Geometry: final body of the model. Coordinates: model frame, mm. Face numbers are marked on the shaded views. A direction names the side the tool comes from. Coordinates: 2 decimals unless noted, no trailing zeros. Loops run counter-clockwise (first coordinate to the right, second up) from the corner with the lowest first, then second, coordinate; pieces in that order, holes last. Notation, with made-up numbers: (60, -5) - (102, -5) arc R9 ccw to (102, 1) - close; hole circle Ø10 at (84, 68.25). An arc over 180 degrees is marked (long way). Return JSON: item names as keys, results as strings.
Solid Edge part; units mm, degrees
sketch "Sketch1" plane through (0, 0, 0) normal (1, 0, 0) x (0, 1, 0)
  line L0 (0, 0) -> (0, 9.5)
  line L1 (0, 9.5) -> (50, 9.5)
  line L2 (50, 9.5) -> (50, 0)
  dimension "D1" = 50
revolve "RevolvedProtrusion1" add sketch "Sketch1" angle 360 about axis through (0, 77.0229, 0) along (0, -1, 0)
sketch "Sketch2" plane through (0, 0, 0) normal (1, 0, 0) x (0, 1, 0)
  line L0 (50, 0) -> (50, 10)
  line L1 (50, 10) -> (66, 10)
  line L2 (66, 10) -> (66, 0)
  dimension "D1" = 50
  dimension "D2" = 66
revolve "RevolvedProtrusion2" add sketch "Sketch2" angle 360 about axis through (0, 158.4797, 0) along (0, -1, 0)
sketch "Sketch3" plane through (0, 0, 0) normal (1, 0, 0) x (0, 1, 0)
  line L0 (66, 0) -> (66, 15)
  line L1 (66, 15) -> (74, 15)
  line L2 (74, 15) -> (74, 0)
  dimension "D1" = 66
  dimension "D2" = 74
revolve "RevolvedProtrusion3" add sketch "Sketch3" angle 360 about axis through (0, 252.6527, 0) along (0, -1, 0)
sketch "Sketch4" plane through (0, 0, 0) normal (1, 0, 0) x (0, 1, 0)
  line L0 (74, 0) -> (74, 20)
  line L1 (74, 20) -> (130, 20)
  line L2 (130, 20) -> (130, 0)
  dimension "D1" = 74
  dimension "D2" = 130
revolve "RevolvedProtrusion4" add sketch "Sketch4" angle 360 about axis through (0, 365.6603, 0) along (0, -1, 0)
sketch "Sketch5" plane through (0, 0, 0) normal (1, 0, 0) x (0, 1, 0)
  line L0 (130, 0) -> (130, 25)
  line L1 (130, 25) -> (140, 25)
  line L2 (140, 25) -> (140, 0)
  dimension "D1" = 130
  dimension "D2" = 140
revolve "RevolvedProtrusion5" add sketch "Sketch5" angle 360 about axis through (0, 524.9007, 0) along (0, -1, 0)
sketch "Sketch6" plane through (0, 0, 0) normal (1, 0, 0) x (0, 1, 0)
  line L0 (140, 0) -> (140, 10)
  line L1 (140, 10) -> (152, 10)
  line L2 (152, 10) -> (152, 0)
  dimension "D1" = 140
  dimension "D2" = 152
revolve "RevolvedProtrusion6" add sketch "Sketch6" angle 360 about axis through (0, 724.416, 0) along (0, -1, 0)
revolve "RevolvedProtrusion7" [suppressed]
revolve "RevolvedProtrusion8" [suppressed]
revolve "RevolvedProtrusion9" [suppressed]
revolve "RevolvedProtrusion10" [suppressed]
revolve "RevolvedProtrusion11" [suppressed]
revolve "RevolvedProtrusion12" [suppressed]
revolve "RevolvedProtrusion13" [suppressed]
revolve "RevolvedProtrusion14" [suppressed]
revolve "RevolvedProtrusion15" [suppressed]
revolve "RevolvedProtrusion16" [suppressed]
revolve "RevolvedProtrusion17" [suppressed]
revolve "RevolvedProtrusion18" [suppressed]
revolve "RevolvedProtrusion19" [suppressed]
revolve "RevolvedProtrusion20" [suppressed]
revolve "RevolvedProtrusion21" [suppressed]
revolve "RevolvedProtrusion22" [suppressed]
revolve "RevolvedProtrusion23" [suppressed]
revolve "RevolvedProtrusion24" [suppressed]
revolve "RevolvedProtrusion25" [suppressed]
sketch "Sketch7" plane through (0, 0, 0) normal (1, 0, 0) x (0, 1, 0)
  line L0 (52.8, 9.5) -> (52.8, 10)
  line L1 (52.8, 10) -> (54, 10)
  line L2 (54, 10) -> (54, 9.5)
  line L3 (54, 9.5) -> (52.8, 9.5)
revolve "RevolvedCutout1" cut sketch "Sketch7" angle 360 about axis through (0, -77.2219, 0) along (0, 1, 0)
revolve "RevolvedCutout2" [suppressed]
revolve "RevolvedCutout3" [suppressed]
revolve "RevolvedCutout4" [suppressed]
sketch "Sketch8" plane through (20, 0, 0) normal (1, 0, 0) x (0, 1, 0)
  line L0 (96, -6) -> (114, -6)
  arc A0 (114, 6) -> (114, -6) centre (114, 0) cw
  line L1 (114, 6) -> (96, 6)
  arc A1 (96, 6) -> (96, -6) centre (96, 0) ccw
extrude "Cutout1" cut sketch "Sketch8" against normal blind 5
extrude "Cutout2" [suppressed]
extrude "Cutout3" [suppressed]
extrude "Cutout4" [suppressed]
extrude "Cutout5" [suppressed]
extrude "Cutout6" [suppressed]
extrude "Cutout7" [suppressed]
extrude "Cutout8" [suppressed]
extrude "Cutout9" [suppressed]
extrude "Cutout10" [suppressed]
extrude "Cutout11" [suppressed]
extrude "Cutout12" [suppressed]
chamfer "Chamfer1" distance 0.5 angle 45 7 edges at (-9.5, 0, 0) (-10, 50, 0) (-15, 66, 0) (-20, 74, 0) (-25, 130, 0) (-25, 140, 0) (-10, 152, 0)
sketch "Sketch9" plane through (0, 0, 0) normal (1, 0, 0) x (0, 1, 0)
  line L0 (80, 19.3) -> (78.25, 19.3)
  line L1 (78.25, 19.3) -> (78.25, 20)
  line L2 (78.25, 20) -> (80, 20)
  line L3 (80, 20) -> (80, 19.3)
sketch3d "WycięciePoKrzywej_1 path"
  arc A0 (0, 74.4999, 20) -> (-17.3205, 74.4999, -10) centre (0, 74.4999, 0)
  arc A1 (-17.3205, 74.4999, -10) -> (17.3205, 74.4999, -10) centre (0, 74.4999, 0)
  arc A2 (17.3205, 74.4999, -10) -> (0, 74.4999, 20) centre (0, 74.4999, 0)
sweep "WycięciePoKrzywej_1" cut profiles "Sketch9" path "WycięciePoKrzywej_1 path"
properties material "Steel"
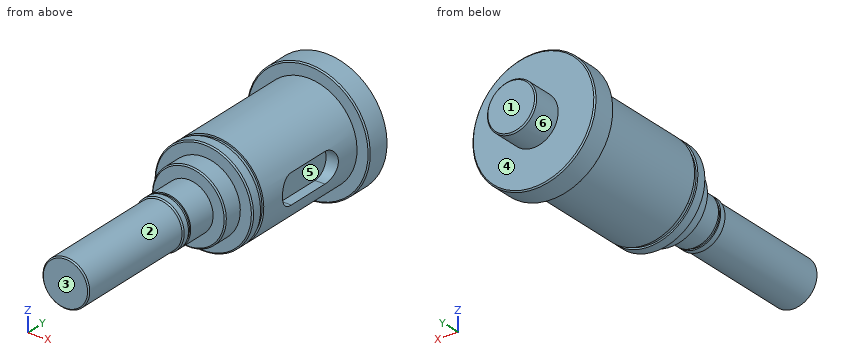
Item 1: Mould query, pull axis Y, two halves, no side actions, for the marked faces 3, 4, 5 and 6. Classes: +Y half, -Y half, draft (parallel to the pull), parting line (faces both ways), or undercut.
Worked out:
{"face 3": "-Y half", "face 4": "+Y half", "face 5": "undercut", "face 6": "draft"}
Item 2: Section query A-A, the plane y = 59.5. Return loops of the section in (x, z), and give its area (3 significant figures).
Worked out:
{"outline": "circle Ø20 at (0, 0)", "area": "314 mm^2"}
Item 3: Section query B-B, the plane y = 35.5. Return loops of the section in (x, z), and give its area (3 significant figures).
Worked out:
{"outline": "circle Ø19 at (0, 0)", "area": "284 mm^2"}
Item 4: First-contact query: pin 1 Ø1.2 at (x, y) = (16.5, 106.5) entering from -Z; pin 2 Ø5 at (x, y) = (-4.5, 106) entering from -Z; pin 3 Ø3.5 at (x, y) = (17, 103.5) entering from +Z. Flat tips, straight axial feed; report the tip coordinate or a pass-through.
Worked out:
{"pin 1": "z = -12.13", "pin 2": "z = -19.9", "pin 3": "z = 12.94"}
Item 5: Ray query, probe 1 along Y at (x, z) = (-2, 21); probe 2 along Y at (x, z) = (-16, -10); probe 3 along X at (y, z) = (101.5, 0.5). Return the intervals inside material, ascending. Write a range as from..to.
Worked out:
{"probe 1": "130..140", "probe 2": "74..140", "probe 3": "-19.99..15"}
Item 6: Reachability of the marked faces 1 and 2 from +Z, -Z, +X, -X, +Y, -Y: full face, straight path, thin tool, end or side. Return the list, or none.
Worked out:
{"face 1": "+Z, -Z, +X, -X, +Y", "face 2": "-Y"}
